from build123d import *

# Parameters (mm, degrees)
SKETCH_3_W      = 170
SKETCH_3_H      = 15
EXTRUDE_3_DEPTH = 5
SKETCH_4_R      = 3.85
SKETCH_4_R_2    = 3.875
SKETCH_4_R_3    = 3.9
SKETCH_4_R_4    = 3.925
SKETCH_4_R_5    = 3.95
SKETCH_4_R_6    = 3.975
SKETCH_4_R_7    = 4
SKETCH_4_R_8    = 4.025
SKETCH_4_R_9    = 4.05
EXTRUDE_4_DEPTH = 10


with BuildPart() as part:
    # 스케치3 → 보스-돌출3 (new body)
    with BuildSketch(Plane(origin=(0, 0, 0), x_dir=(1, 0, 0), z_dir=(0, 1, 0))):
        Rectangle(SKETCH_3_W, SKETCH_3_H)
    extrude(amount=EXTRUDE_3_DEPTH)

    # 스케치4 → 보스-돌출4 (add)
    with BuildSketch(Plane(origin=(0, 5, 0), x_dir=(1, 0, 0), z_dir=(0, 1, 0))):
        with Locations(Location((-80, 0, 0), (0, 0, 90))):
            Circle(SKETCH_4_R)
        with Locations(Location((-60, 0, 0), (0, 0, 90))):
            Circle(SKETCH_4_R_2)
        with Locations(Location((-40, 0, 0), (0, 0, 90))):
            Circle(SKETCH_4_R_3)
        with Locations(Location((-20, 0, 0), (0, 0, 90))):
            Circle(SKETCH_4_R_4)
        with Locations(Location((0, 0, 0), (0, 0, 90))):
            Circle(SKETCH_4_R_5)
        with Locations(Location((20, 0, 0), (0, 0, 90))):
            Circle(SKETCH_4_R_6)
        with Locations(Location((40, 0, 0), (0, 0, 90))):
            Circle(SKETCH_4_R_7)
        with Locations(Location((60, 0, 0), (0, 0, 90))):
            Circle(SKETCH_4_R_8)
        with Locations(Location((80, 0, 0), (0, 0, 90))):
            Circle(SKETCH_4_R_9)
    extrude(amount=EXTRUDE_4_DEPTH)


solid = part.part
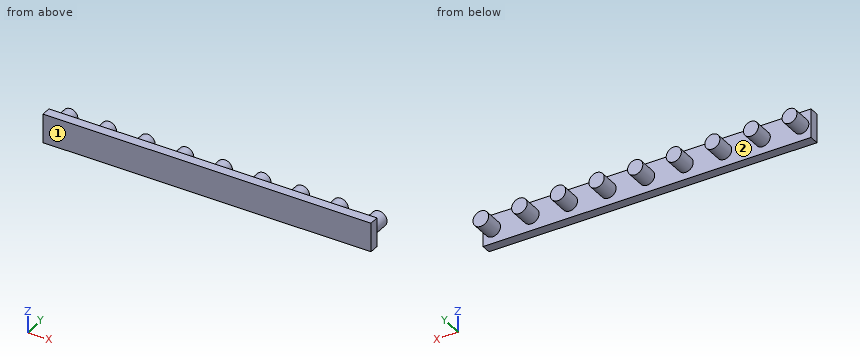
Geometry check sheet. Reference: the model listing, model coordinates, mm. Face numbers are marked on the shaded views. A direction names the side the tool comes from. Round coordinates to 2 decimals unless told otherwise and drop trailing zeros. Loops run counter-clockwise (first coordinate to the right, second up) from the corner with the lowest first, then second, coordinate; pieces in that order, holes last. Notation, with made-up numbers: (19.5, 55) -> (46.5, 55) arc R25 ccw to (46.5, 68) -> close; hole circle Ø4 at (-19, 17.25). An arc over 180 degrees is marked (long way). Answer as a JSON object with one key per item and string values. Group by question number.
Item 1: Cross-section at C-C, the plane x = -20. Record the cut outline in (y, z) (3 decimals).
Item 2: Thickness scan on line 1 along Y through (x, z) = (-8.5, 1.5); line 2 along Z through (x, y) = (-1, 9); line 3 along Z through (x, y) = (61.5, 11). Record the ranges inside material, lowest first.
Item 3: Set-up check for the marked faces 1 and 2: record each of +Z, -Z, +X, -X, +Y, -Y from which the full face is reachable in a straight line by a thin tool's end or side.
Item 4: Depth check by flat-ended pin: pin 1 Ø7.5 at (x, z) = (32, -1.5) entering from +Y; pin 2 Ø1 at (x, y) = (-37, 8.5) entering from -Z. Enter the tip coordinate at first touch or a pass-through.
Item 5: Cross-section at A-A, the plane y = 7.25. Count the separate pieces of the cut face and the enclosed holes in it, plus the area to 3 significant figures.
Item 6: Cross-section at B-B, the plane x = 0. Record the cut outline in (y, z).
Determined:
{
 "1": {"outline": "(0, -7.5) -> (5, -7.5) -> (5, -3.925) -> (15, -3.925) -> (15, 3.925) -> (5, 3.925) -> (5, 7.5) -> (0, 7.5) -> close"},
 "2": {"line 1": "y = 0 to 5", "line 2": "z = -3.82 to 3.82", "line 3": "z = -3.74 to 3.74"},
 "3": {"face 1": "+Z, -Z, +X, -X, -Y", "face 2": "+Y"},
 "4": {"pin 1": "stops at y = 5", "pin 2": "stops at z = -2.99"},
 "5": {"separate pieces": "9", "enclosed holes": "0", "area": "441 mm²"},
 "6": {"outline": "(0, -7.5) -> (5, -7.5) -> (5, -3.95) -> (15, -3.95) -> (15, 3.95) -> (5, 3.95) -> (5, 7.5) -> (0, 7.5) -> close"}
}
